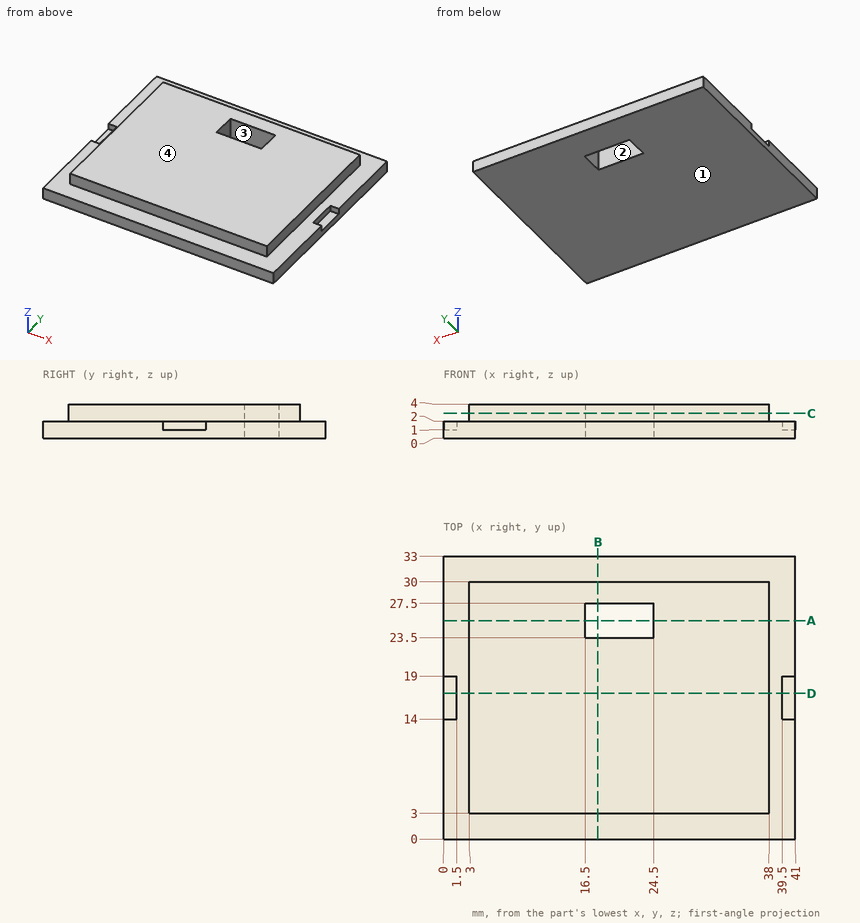
Study the drawing (mm; zero at the part's minimum x, y, z) and answer. A direction names the side the tool comes from. Coordinates: 2 decimals unless noted, no trailing zeros. Loops run counter-clockwise (first coordinate to the right, second up) from the corner with the lowest first, then second, coordinate; pieces in that order, holes last. Notation, with made-up numbers: (-35.5, -12) -> (7.5, -12) arc R10 cw to (7.5, 7) -> close; hole circle Ø1 at (26, 14.5). An arc over 180 degrees is marked (long way). Write each question's results on one line, items separated by ' | '. Start each with the question number.
1) Consider line 1 along Y through (x, z) = (23, 2.1); line 2 along X through (y, z) = (27, 3.15); line 3 along X through (y, z) = (15.5, 2.6). Determine where each line is inside the solid, lowest interval first.
2) The mould has two halves that part along Y. Classify the marked faces 1 and 2: pulls with the +Y half, pulls with the -Y half, needs draft (parallel to the pull), parting line crosses it, or undercut.
3) Find section B-B on x = 18. Determine the outline of the cut face in (y, z).
4) For the marked faces 3 and 4, determine the directions among +Z, -Z, +X, -X, +Y, -Y from which every point of the face is accessible in a straight line to the end or side of a thin tool.
5) Flat-ended cylindrical pins translate along their axes: P1, Ø0.8, axis at y = 17, z = 1.5, coming from the -X side; P2, Ø4, axis at x = 19.5, y = 23.5, coming from the -Z side; P3, Ø0.6, axis at y = 14.5, z = 3, coming from the +X side; P4, Ø1, axis at y = 8, z = 3, coming from the -X side. Find the tip coordinate at first contact, or state that the pin passes through.
6) Find section D-D on y = 17. Determine the outline of the cut face in (x, z).
7) Find section C-C on z = 2.9. Determine the outline of the cut face in (x, y), then the cut area to 3 significant figures.
8) Find section A-A on y = 25.5. Determine the outline of the cut face in (x, z).
Response values:
1) line 1: y = 3 to 23.5, 27.5 to 30 | line 2: x = 3 to 16.5, 24.5 to 38 | line 3: x = 3 to 38
2) face 1: needs draft | face 2: undercut
3) outline: (0, 0) -> (23.5, 0) -> (23.5, 4) -> (3, 4) -> (3, 2) -> (0, 2) -> close; (27.5, 0) -> (33, 0) -> (33, 2) -> (30, 2) -> (30, 4) -> (27.5, 4) -> close
4) face 3: +Z, -Z | face 4: +Z, +X, -X, +Y, -Y
5) P1: stops at x = 1.5 | P2: stops at z = 0 | P3: stops at x = 38 | P4: stops at x = 3
6) outline: (0, 0) -> (41, 0) -> (41, 1) -> (39.5, 1) -> (39.5, 2) -> (38, 2) -> (38, 4) -> (3, 4) -> (3, 2) -> (1.5, 2) -> (1.5, 1) -> (0, 1) -> close
7) outline: (3, 3) -> (38, 3) -> (38, 30) -> (3, 30) -> close; hole (16.5, 23.5) -> (24.5, 23.5) -> (24.5, 27.5) -> (16.5, 27.5) -> close | area: 913 mm^2
8) outline: (0, 0) -> (16.5, 0) -> (16.5, 4) -> (3, 4) -> (3, 2) -> (0, 2) -> close; (24.5, 0) -> (41, 0) -> (41, 2) -> (38, 2) -> (38, 4) -> (24.5, 4) -> close
